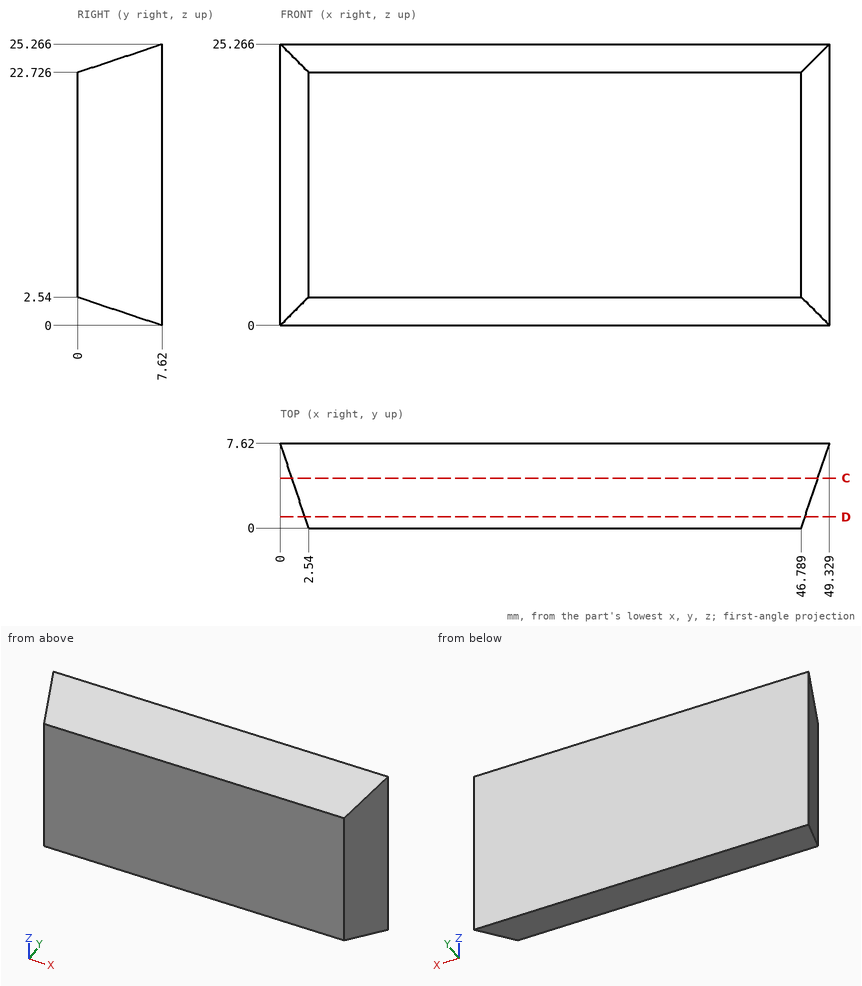
Check sheet for the drawn part. Datum: minimum x, y, z corner. Units: mm. Round coordinates to 2 decimals unless told otherwise and drop trailing zeros. Order: outer loops, then holes, each group sorted by start corner. A loop starts at its lowest first (then second) coordinate and runs counter-clockwise, first axis right, second up.
(1) Go/stop test with flat-tipped pins: P1, Ø1.5, axis at x = 9, y = 4, coming from the -Z side; P2, Ø1, axis at x = 30.5, y = 2.5, coming from the -Z side; P3, Ø2, axis at x = 23, y = 1, coming from the +Z side. Record where each tip stops, or that it passes through.
(2) Cross-section at D-D, the plane y = 1. Enter the section's corners in (x, z), and give its area (3 significant figures).
(3) Cross-section at C-C, the plane y = 4.5. Enter the section's corners in (x, z).
(4) Scan lines: probe 1 along Z at (x, y) = (34, 0.5); probe 2 along X at (y, z) = (2.5, 11.5); probe 3 along X at (y, z) = (2, 16) (1 decimal). Record each from-to range of solid material in increasing order.
Check sheet entries:
1. P1: stops at z = 0.96
1. P2: stops at z = 1.54
1. P3: stops at z = 23.39
2. outline: (2.21, 2.21) - (47.12, 2.21) - (47.12, 23.06) - (2.21, 23.06) - close
2. area: 937 mm2
3. outline: (1.04, 1.04) - (48.29, 1.04) - (48.29, 24.23) - (1.04, 24.23) - close
4. probe 1: z = 2.37 to 22.89
4. probe 2: x = 1.71 to 47.62
4. probe 3: x = 1.9 to 47.5
